Can you work these out from the model? Positions are in its coordinate system, mm. Face numbers are marked on the shaded views. A direction names the side the tool comes from. Coordinates: 2 decimals unless noted, no trailing zeros. Loops run counter-clockwise (first coordinate to the right, second up) from the corner with the lowest first, then second, coordinate; pieces in that order, holes last.
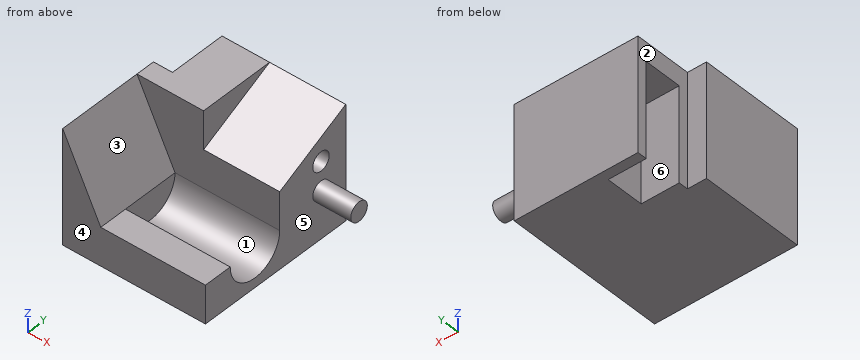
```python
from build123d import *

# Parameters (mm, degrees)
F0_W      = 75
F0_H      = 85
F1_DEPTH  = 60
F2_R      = 5
F3_DEPTH  = 20
F4_R      = 5
F5_DEPTH  = 30
F6_W      = 10
F6_H      = 30
F7_DEPTH  = 60.001
F9_DEPTH  = 45
F11_DEPTH = 40
F12_W     = 45
F12_H     = 40
F13_DEPTH = 55
F14_R     = 15
F15_DEPTH = 55
F16_W     = 20
F16_H     = 20
F17_DEPTH = 50


with BuildPart() as f1:
    # F0 (on Top) → F1 (new body)
    with BuildSketch(Plane.XY):
        with Locations((37.5, 42.5)):
            Rectangle(F0_W, F0_H)
    extrude(amount=F1_DEPTH)

    # F2 (on face) → F3 (join)
    with BuildSketch(Plane.YZ.offset(75)):
        with Locations((70, 25)):
            Circle(F2_R)
    extrude(amount=F3_DEPTH)

    # F4 (on face) → F5 (cut)
    with BuildSketch(Plane.YZ.offset(75)):
        with Locations((70, 40)):
            Circle(F4_R)
    extrude(amount=-F5_DEPTH, mode=Mode.SUBTRACT)

    # F6 (on face) → F7 (cut, through all)
    with BuildSketch(Plane.XY.offset(60)):
        with Locations((5, 70)):
            Rectangle(F6_W, F6_H)
    extrude(amount=-F7_DEPTH, mode=Mode.SUBTRACT)

    # F8 (on face) → F9 (cut)
    with BuildSketch(Plane.XZ):
        Polygon((20, 60), (0, 60), (20, 20), align=None)
    extrude(amount=-F9_DEPTH, mode=Mode.SUBTRACT)

    # F10 (on face) → F11 (cut)
    with BuildSketch(Plane.YZ.offset(75)):
        Polygon((45, 40), (85, 60), (45, 60), align=None)
    extrude(amount=-F11_DEPTH, mode=Mode.SUBTRACT)

    # F12 (on face) → F13 (cut)
    with BuildSketch(Plane.YZ.offset(75)):
        with Locations((22.5, 40)):
            Rectangle(F12_W, F12_H)
    extrude(amount=-F13_DEPTH, mode=Mode.SUBTRACT)

    # F14 (on face) → F15 (cut, through all)
    with BuildSketch(Plane.YZ.offset(75)):
        with Locations((30, 20)):
            Circle(F14_R)
    extrude(amount=-F15_DEPTH, mode=Mode.SUBTRACT)

    # F16 (on face) → F17 (cut)
    with BuildSketch(Plane(origin=(0, 0, 0), x_dir=(1, 0, 0), z_dir=(0, 0, -1))):
        with Locations((20, -70)):
            Rectangle(F16_W, F16_H)
    extrude(amount=-F17_DEPTH, mode=Mode.SUBTRACT)


solid = f1.part
```
Item 1: Suppose I cut it at D-D, the plane y = 30. Please give me the cut outline in (x, z), plus the area to 4 significant figures.
Results are:
outline: (0, 0) - (75, 0) - (75, 5) - (20, 5) - (20, 20) - (0, 60) - close
area: 1,075 mm2
Item 2: I'm going to push flat-ended pins straight in: P1, Ø4.5, axis at y = 28.5, z = 10, coming from the +X side; P2, Ø8, axis at y = 34, z = 46.5, coming from the -X side; P3, Ø1.5, axis at x = 26, y = 40, coming from the +Z side; P4, Ø15, axis at y = 76.5, z = 38.5, coming from the -X side. Where does each tip first touch, or does it pass through?
Results are:
P1: stops at x = 20
P2: stops at x = 0
P3: stops at z = 9.54
P4: stops at x = 10
Item 3: Suppose I cut it at A-A, the plane x = 49. Please give me the cut outline in (y, z).
Results are:
outline: (0, 0) - (85, 0) - (85, 60) - (45, 40) - (45, 20) arc R15 cw to (15, 20) - (0, 20) - close; hole circle Ø10 at (70, 40)
Item 4: I need wall thicknesses on line 1 along Y through (x, z) = (29, 45); line 2 along X through (y, z) = (69, 7.5); line 3 along Y through (x, z) = (20.5, 3). Which ranges of each line are inside material? Lowest first, please.
Results are:
line 1: y = 45 to 60, 80 to 85
line 2: x = 30 to 75
line 3: y = 0 to 60, 80 to 85
Item 5: Suppose I cut it at C-C, the plane z = 25. Please give me the cut outline in (x, y), plus the area to 3 significant figures.
Results are:
outline: (0, 0) - (17.5, 0) - (17.5, 45) - (75, 45) - (75, 65) - (95, 65) - (95, 75) - (75, 75) - (75, 85) - (10, 85) - (10, 80) - (30, 80) - (30, 60) - (10, 60) - (10, 55) - (0, 55) - close
area: 3,290 mm2
Item 6: Suppose I cut it at B-B, the plane x = 18. Please give me the cut outline in (y, z).
Results are:
outline: (0, 0) - (60, 0) - (60, 50) - (80, 50) - (80, 0) - (85, 0) - (85, 60) - (45, 60) - (45, 24) - (0, 24) - close
Item 7: We'd pull the mould along Y, two halves only. Please class the marked faces 4, 5 and 6: +Y half, -Y half, draft (parallel to the pull), parting line (faces both ways), or undercut.
Results are:
face 4: -Y half
face 5: draft
face 6: undercut
Item 8: On a 3-axis mill with a long thin cutter (end or side, diameter ignored), from which of +Z, -Z, +X, -X, +Y, -Y can I reach the whole of each face in a straight line? I mean the marked faces 1, 2 and 3. Say none if no direction works.
Results are:
face 1: +Z, +X
face 2: +Z, -Z, -X, +Y
face 3: +Z, +X, -Y
